Answer from the drawing. Dimensions are ordinates in mm from the lowest x, y and z of the part. Give positions to 0.01 mm unless a question says otherwise; leave off trailing zeros. Loops run counter-clockwise (first coordinate to the right, second up) from the corner with the lowest first, then second, coordinate; pieces in that order, holes last.
Item 1: Section B-B, the plane z = 3.5 is taken. Give the vertices of the cut face in (x, y), and give its area (4 significant figures).
Item 2: Each of these flat-tipped pins is pushed along its axis until it touches: pin 1 Ø3.5 at (y, z) = (2.5, 2.5) entering from +X; pin 2 Ø1.8 at (x, z) = (6.5, 3.5) entering from -Y; pin 3 Ø5 at (x, z) = (25, 9) entering from +Y. Where does it stop, or does it pass through?
Item 3: Consider line 1 along Z through (x, y) = (6.5, 1.4); line 2 along X through (y, z) = (2.35, 10.5); line 3 along Y through (x, z) = (121.5, 13.5). Determine where each line is inside the solid, lowest interval first.
Item 4: Section C-C, the plane x = 103.5 is taken. Give the vertices of the cut face in (y, z).
Item 5: Section A-A, the plane x = 6.5 is taken. Give the vertices of the cut face in (y, z), and give its area (3 significant figures).
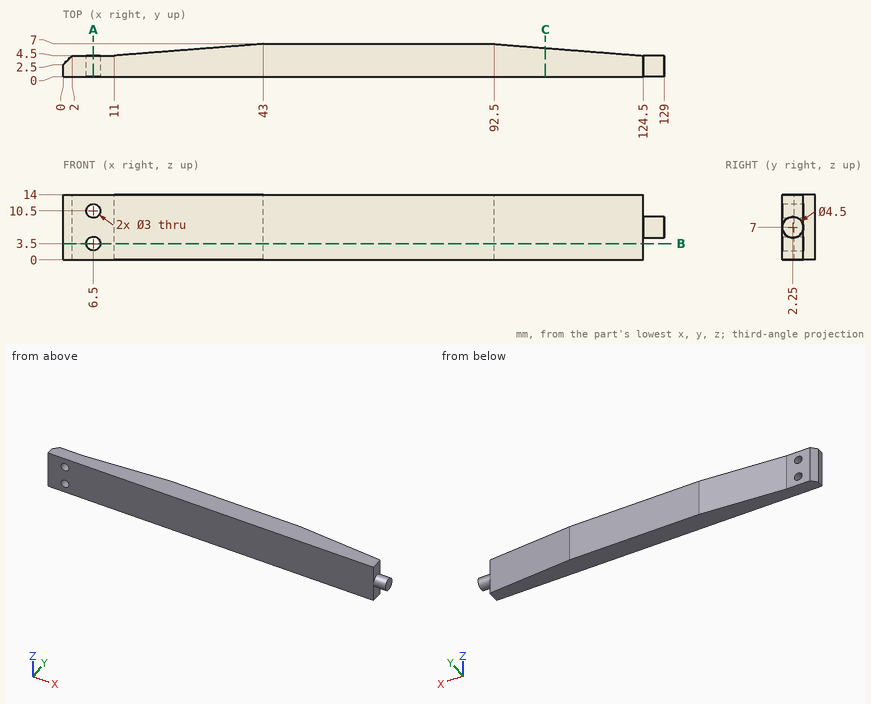
Worked answers:
1. outline: (0, 0) - (5, 0) - (5, 4.5) - (2, 4.5) - (0, 2.5) - close; (8, 0) - (124.5, 0) - (124.5, 4.5) - (92.5, 7) - (43, 7) - (11, 4.5) - (8, 4.5) - close
1. area: 748.5 mm2
2. pin 1: stops at x = 124.5
2. pin 2: passes through
2. pin 3: stops at y = 5.79
3. line 1: z = 0 to 2, 5 to 9, 12 to 14
3. line 2: x = 0 to 5, 8 to 124.5
3. line 3: y = 0 to 4.73
4. outline: (0, 0) - (6.14, 0) - (6.14, 14) - (0, 14) - close
5. outline: (0, 0) - (4.5, 0) - (4.5, 2) - (0, 2) - close; (0, 5) - (4.5, 5) - (4.5, 9) - (0, 9) - close; (0, 12) - (4.5, 12) - (4.5, 14) - (0, 14) - close
5. area: 36.0 mm2
